Part print with two shaded views. Sizes in mm from the minimum x, y, z corner. Coordinates: 2 decimals unless noted, no trailing zeros. Loops run counter-clockwise (first coordinate to the right, second up) from the corner with the lowest first, then second, coordinate; pieces in that order, holes last.
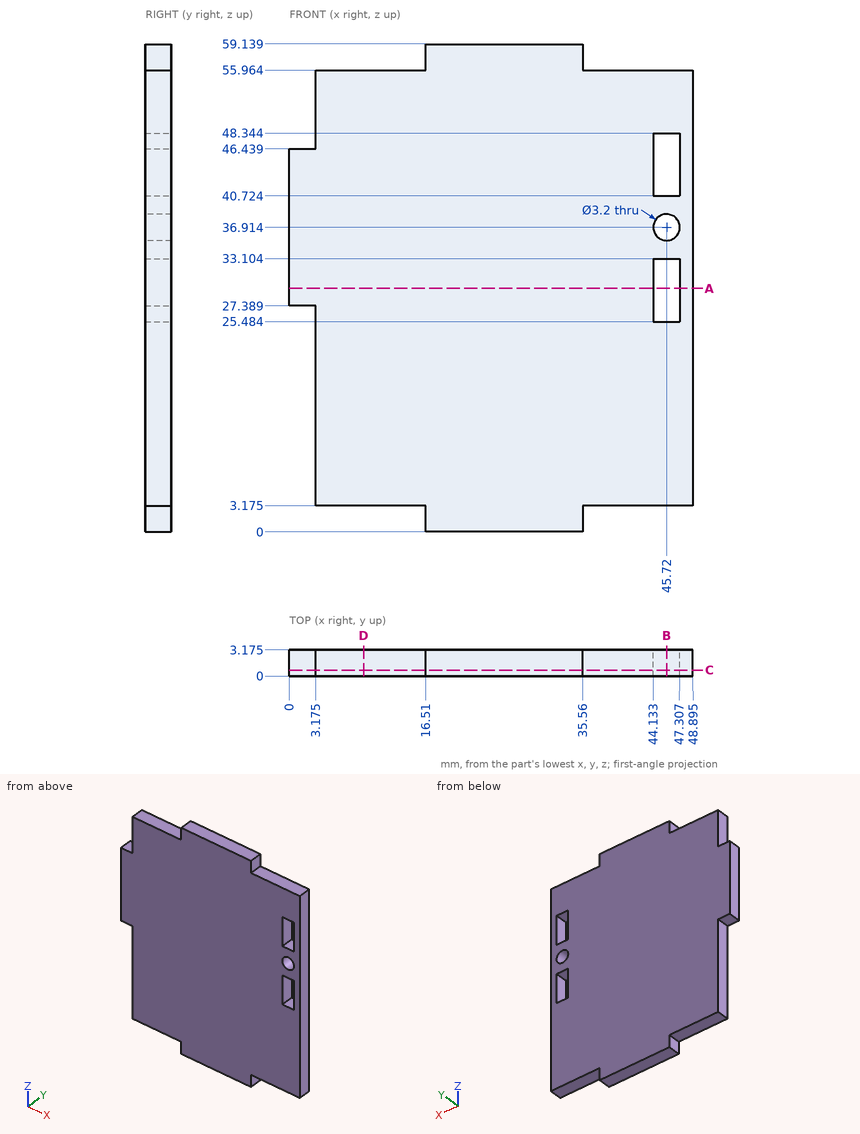
Q1. Drill centre lines: line 1 (Z direction, x = 45.72, y = 0.8) (1 decimal); line 2 (X direction, y = 2.2, z = 26.5) (1 decimal); line 3 (X direction, y = 0.8, z = 46) (1 decimal). Where is each one in solid material? Low to high.
Answers:
line 1: z = 3.2 to 25.5, 33.1 to 35.3, 38.5 to 40.7, 48.3 to 56
line 2: x = 3.2 to 44.1, 47.3 to 48.9
line 3: x = 0 to 44.1, 47.3 to 48.9
Q2. Slice it at A-A (z = 29.5). List the corners of the cut face in (x, y) (1 decimal).
Answers:
outline: (0, 0) - (44.1, 0) - (44.1, 3.2) - (0, 3.2) - close; (47.3, 0) - (48.9, 0) - (48.9, 3.2) - (47.3, 3.2) - close
Q3. Slice it at C-C (y = 0.7). List the corners of the cut face in (x, z) (1 decimal), and give its area (3 significant figures).
Answers:
outline: (0, 27.4) - (3.2, 27.4) - (3.2, 3.2) - (16.5, 3.2) - (16.5, 0) - (35.6, 0) - (35.6, 3.2) - (48.9, 3.2) - (48.9, 56) - (35.6, 56) - (35.6, 59.1) - (16.5, 59.1) - (16.5, 56) - (3.2, 56) - (3.2, 46.4) - (0, 46.4) - close; hole (44.1, 25.5) - (47.3, 25.5) - (47.3, 33.1) - (44.1, 33.1) - close; hole circle Ø3.2 at (45.7, 36.9); hole (44.1, 40.7) - (47.3, 40.7) - (47.3, 48.3) - (44.1, 48.3) - close
area: 2,540 mm2
Q4. Flat gauge pins, fed straight in: P1, Ø1, axis at x = 11, y = 1.5, coming from the +Z side; P2, Ø1.6, axis at x = 42.5, y = 2, coming from the -Z side (1 decimal); P3, Ø1, axis at x = 1, y = 2, coming from the +Z side. Where does each tip first touch, or does it go through?
Answers:
P1: stops at z = 55.96
P2: stops at z = 3.2
P3: stops at z = 46.44
Q5. Slice it at D-D (x = 9). List the corners of the cut face in (y, z) (1 decimal).
Answers:
outline: (0, 3.2) - (3.2, 3.2) - (3.2, 56) - (0, 56) - close
Q6. Slice it at B-B (x = 45.72). List the corners of the cut face in (y, z) (1 decimal).
Answers:
outline: (0, 3.2) - (3.2, 3.2) - (3.2, 25.5) - (0, 25.5) - close; (0, 33.1) - (3.2, 33.1) - (3.2, 35.3) - (0, 35.3) - close; (0, 38.5) - (3.2, 38.5) - (3.2, 40.7) - (0, 40.7) - close; (0, 48.3) - (3.2, 48.3) - (3.2, 56) - (0, 56) - close
